from build123d import *

# Parameters (mm, degrees)
SKETCH_W       = 25
SKETCH_H       = 25
PAD_DEPTH      = 15
SKETCH002_W    = 21
SKETCH002_H    = 21
SKETCH001_W    = 23
SKETCH001_H    = 23
SKETCH004_W    = 25
SKETCH004_H    = 25
PAD001_DEPTH   = 20
CYLINDER_R     = 10
CYLINDER_DEPTH = 20


with BuildPart() as body:
    # Sketch → Pad (new body)
    with BuildSketch(Plane.XY):
        Rectangle(SKETCH_W, SKETCH_H)
    extrude(amount=PAD_DEPTH)

    # Sketch002 (on Face5 of Pad) → SubtractiveLoft section 0
    with BuildSketch(Plane(origin=(0, 0, 0), x_dir=(1, 0, 0), z_dir=(0, 0, -1))):
        Rectangle(SKETCH002_W, SKETCH002_H)
    # Sketch001 (on Face6 of Pad) → SubtractiveLoft section 1
    with BuildSketch(Plane.XY.offset(15)):
        Rectangle(SKETCH001_W, SKETCH001_H)
    loft(mode=Mode.SUBTRACT)


with BuildPart() as body001:
    # Sketch004 → Pad001 (new body)
    with BuildSketch(Plane.XY):
        Rectangle(SKETCH004_W, SKETCH004_H)
    extrude(amount=PAD001_DEPTH)

    # Boolean: cut Body
    add(body.part, mode=Mode.SUBTRACT)

    # Cylinder → Cylinder (cut)
    with BuildSketch(Plane.XY):
        Circle(CYLINDER_R)
    extrude(amount=CYLINDER_DEPTH, mode=Mode.SUBTRACT)


solid = body001.part
Source: CAD feature listing. Evaluate the final solid. Frame: model axes, mm. Give positions to 0.01 mm unless a question says otherwise; leave off trailing zeros. Order: outer loops, then holes, each group sorted by start corner. A loop starts at its lowest first (then second) coordinate and runs counter-clockwise, first axis right, second up. Notation, with made-up numbers: (83.25, 75) -> (113.25, 75) arc R36 ccw to (113.25, 109) -> close; hole circle Ø11 at (26.25, -7). An arc over 180 degrees is marked (long way). Write item = value, one per line.
Item 1: Ray query, probe 1 along Y at (x, z) = (-2.25, 8.5); probe 2 along Y at (x, z) = (0, 6.5); probe 3 along X at (y, z) = (7.25, 4). Return the intervals inside material, ascending.
Check result:
probe_1 = -11.07 to -9.74, 9.74 to 11.07
probe_2 = -10.93 to -10, 10 to 10.93
probe_3 = -10.77 to -6.89, 6.89 to 10.77
Item 2: Contact query for flat-ended pins moving along their axis: pin 1 (4 mm diameter, centred on y = -5, z = 13.5, fed in from -X); pin 2 (3 mm diameter, centred on y = -5, z = 10.5, fed in from -X); pin 3 (2 mm diameter, centred on y = 9, z = 6, fed in from -X); pin 4 (2 mm diameter, centred on x = -4, z = 4.5, fed in from +Y). Output: stop coordinate, or through.
Check result:
pin_1 = -12.5
pin_2 = -11.3
pin_3 = -10.97
pin_4 = 10.87
Item 3: Mould query, pull axis Y, two halves, no side actions, for faces 1 (the face through (0, 12.5, 17)), 2 (the face through (-1, -12, 15)), 3 (the face through (0, -12.5, 17)), 4 (the face through (-2.17, -9.76, 9.86)). Classes: +Y half, -Y half, draft (parallel to the pull), parting line (faces both ways), or undercut.
Check result:
face_1 = +Y half
face_2 = draft
face_3 = -Y half
face_4 = undercut
Item 4: Section query A-A (z = 16.25). Output: boundary loops of the cut face in (x, y), then the cut area to 3 significant figures.
Check result:
outline = (-12.5, -12.5) -> (12.5, -12.5) -> (12.5, 12.5) -> (-12.5, 12.5) -> close; hole circle Ø20 at (0, 0)
area = 311 mm²
